Input: part model. Units: mm. Frame: model coordinates. A direction names the side the tool comes from. Give positions to 0.01 mm unless a question says otherwise; leave off trailing zeros. Loops run counter-clockwise (first coordinate to the right, second up) from the corner with the lowest first, then second, coordinate; pieces in that order, holes last. Notation, with made-up numbers: M -22,0 L 20,0 A23 cw 20,17 Z; hole C 0.25,-29 d5. An arc over 180 degrees is marked long. Answer as a JSON object with one key per item and string values. Group by question number.
```python
from build123d import *

# Parameters (mm, degrees)
F1_DEPTH = 5.08
F3_DEPTH = 25.4
F4_R     = 2.54
F5_R     = 1.524


with BuildPart() as f1:
    # F0 (on Top) → F1 (new body)
    with BuildSketch(Plane.XY):
        with BuildLine():
            ThreePointArc((-13.7862916745, 2.2581102419), (-1.1327853518, -13.9239971756), (13.97, 0))
            ThreePointArc((13.97, 0), (13.9239971756, 1.1327853518), (13.7862916745, 2.2581102419))
            ThreePointArc((13.7862916745, 2.2581102419), (9.0447526202, 10.646753028), (0, 13.97))
            ThreePointArc((0, 13.97), (-9.0447526202, 10.646753028), (-13.7862916745, 2.2581102419))
        make_face()
        with BuildLine():
            Line((-6.6675, 45.72), (-13.7862916745, 2.2581102419))
            ThreePointArc((-13.7862916745, 2.2581102419), (-9.0447526202, 10.646753028), (0, 13.97))
            Line((0, 13.97), (-1.5875, 13.97))
            Line((-1.5875, 13.97), (-1.5875, 45.72))
            Line((-1.5875, 45.72), (-6.6675, 45.72))
        make_face()
        with BuildLine():
            ThreePointArc((0, 13.97), (9.0447526202, 10.646753028), (13.7862916745, 2.2581102419))
            Line((13.7862916745, 2.2581102419), (6.6675, 45.72))
            Line((6.6675, 45.72), (1.5875, 45.72))
            Line((1.5875, 45.72), (1.5875, 13.97))
            Line((1.5875, 13.97), (0, 13.97))
        make_face()
    extrude(amount=F1_DEPTH)

    # F2 (on face) → F3 (cut)
    with BuildSketch(Plane.XY.offset(5.08)):
        with BuildLine():
            Line((-3.7422612851, 9.0346179484), (-1.9134612851, 9.0346179484))
            ThreePointArc((-1.9134612851, 9.0346179484), (-4.4421127462, 10.7242088375), (-5.0354181665, 7.741461067))
            Line((-5.0354181665, 7.741461067), (-3.7422612851, 9.0346179484))
        make_face()
        with BuildLine():
            ThreePointArc((-5.0354181665, 7.741461067), (-3.042409824, 7.3450270594), (-1.9134612851, 9.0346179484))
            Line((-1.9134612851, 9.0346179484), (-3.7422612851, 9.0346179484))
            Line((-3.7422612851, 9.0346179484), (-5.0354181665, 7.741461067))
        make_face()
        with BuildLine():
            Line((3.7422612851, 9.0346179484), (5.0354181665, 7.741461067))
            ThreePointArc((5.0354181665, 7.741461067), (5.4318521742, 8.3347664873), (5.5710612851, 9.0346179484))
            ThreePointArc((5.5710612851, 9.0346179484), (3.7422612851, 10.8634179484), (1.9134612851, 9.0346179484))
            Line((1.9134612851, 9.0346179484), (3.7422612851, 9.0346179484))
        make_face()
        with BuildLine():
            ThreePointArc((1.9134612851, 9.0346179484), (3.042409824, 7.3450270594), (5.0354181665, 7.741461067))
            Line((5.0354181665, 7.741461067), (3.7422612851, 9.0346179484))
            Line((3.7422612851, 9.0346179484), (1.9134612851, 9.0346179484))
        make_face()
        with BuildLine():
            Line((7.741461067, 5.0354181665), (9.0346179484, 3.7422612851))
            Line((9.0346179484, 3.7422612851), (9.0346179484, 1.9134612851))
            ThreePointArc((9.0346179484, 1.9134612851), (10.3277748299, 2.4491044037), (10.8634179484, 3.7422612851))
            ThreePointArc((10.8634179484, 3.7422612851), (9.7344694095, 5.4318521742), (7.741461067, 5.0354181665))
        make_face()
        with BuildLine():
            Line((9.0346179484, 1.9134612851), (9.0346179484, 3.7422612851))
            Line((9.0346179484, 3.7422612851), (7.741461067, 5.0354181665))
            ThreePointArc((7.741461067, 5.0354181665), (7.3450270594, 3.042409824), (9.0346179484, 1.9134612851))
        make_face()
        with BuildLine():
            ThreePointArc((10.8634179484, -3.7422612851), (10.3277748299, -2.4491044037), (9.0346179484, -1.9134612851))
            Line((9.0346179484, -1.9134612851), (9.0346179484, -3.7422612851))
            Line((9.0346179484, -3.7422612851), (7.741461067, -5.0354181665))
            ThreePointArc((7.741461067, -5.0354181665), (9.7344694095, -5.4318521742), (10.8634179484, -3.7422612851))
        make_face()
        with BuildLine():
            Line((9.0346179484, -3.7422612851), (9.0346179484, -1.9134612851))
            ThreePointArc((9.0346179484, -1.9134612851), (7.3450270594, -3.042409824), (7.741461067, -5.0354181665))
            Line((7.741461067, -5.0354181665), (9.0346179484, -3.7422612851))
        make_face()
        with BuildLine():
            ThreePointArc((5.5710612851, -9.0346179484), (5.4318521742, -8.3347664873), (5.0354181665, -7.741461067))
            Line((5.0354181665, -7.741461067), (3.7422612851, -9.0346179484))
            Line((3.7422612851, -9.0346179484), (1.9134612851, -9.0346179484))
            ThreePointArc((1.9134612851, -9.0346179484), (3.7422612851, -10.8634179484), (5.5710612851, -9.0346179484))
        make_face()
        with BuildLine():
            Line((3.7422612851, -9.0346179484), (5.0354181665, -7.741461067))
            ThreePointArc((5.0354181665, -7.741461067), (3.042409824, -7.3450270594), (1.9134612851, -9.0346179484))
            Line((1.9134612851, -9.0346179484), (3.7422612851, -9.0346179484))
        make_face()
        with BuildLine():
            ThreePointArc((-5.0354181665, -7.741461067), (-4.4421127462, -10.7242088375), (-1.9134612851, -9.0346179484))
            Line((-1.9134612851, -9.0346179484), (-3.7422612851, -9.0346179484))
            Line((-3.7422612851, -9.0346179484), (-5.0354181665, -7.741461067))
        make_face()
        with BuildLine():
            Line((-3.7422612851, -9.0346179484), (-1.9134612851, -9.0346179484))
            ThreePointArc((-1.9134612851, -9.0346179484), (-3.042409824, -7.3450270594), (-5.0354181665, -7.741461067))
            Line((-5.0354181665, -7.741461067), (-3.7422612851, -9.0346179484))
        make_face()
        with BuildLine():
            Line((-9.0346179484, -3.7422612851), (-7.741461067, -5.0354181665))
            ThreePointArc((-7.741461067, -5.0354181665), (-7.3450270594, -4.4421127462), (-7.2058179484, -3.7422612851))
            ThreePointArc((-7.2058179484, -3.7422612851), (-7.741461067, -2.4491044037), (-9.0346179484, -1.9134612851))
            Line((-9.0346179484, -1.9134612851), (-9.0346179484, -3.7422612851))
        make_face()
        with BuildLine():
            ThreePointArc((-9.0346179484, -1.9134612851), (-10.7242088375, -4.4421127462), (-7.741461067, -5.0354181665))
            Line((-7.741461067, -5.0354181665), (-9.0346179484, -3.7422612851))
            Line((-9.0346179484, -3.7422612851), (-9.0346179484, -1.9134612851))
        make_face()
        with BuildLine():
            Line((-9.0346179484, 3.7422612851), (-7.741461067, 5.0354181665))
            ThreePointArc((-7.741461067, 5.0354181665), (-10.7242088375, 4.4421127462), (-9.0346179484, 1.9134612851))
            Line((-9.0346179484, 1.9134612851), (-9.0346179484, 3.7422612851))
        make_face()
        with BuildLine():
            ThreePointArc((-7.2058179484, 3.7422612851), (-7.3450270594, 4.4421127462), (-7.741461067, 5.0354181665))
            Line((-7.741461067, 5.0354181665), (-9.0346179484, 3.7422612851))
            Line((-9.0346179484, 3.7422612851), (-9.0346179484, 1.9134612851))
            ThreePointArc((-9.0346179484, 1.9134612851), (-7.741461067, 2.4491044037), (-7.2058179484, 3.7422612851))
        make_face()
    extrude(amount=-F3_DEPTH, mode=Mode.SUBTRACT)

    # F4
    f4_edges = [f1.edges().sort_by_distance(p)[0] for p in [
        (1.5875, 45.72, 2.54),
        (-1.5875, 45.72, 2.54),
        (-6.6675, 45.72, 2.54),
        (6.6675, 45.72, 2.54),
    ]]
    fillet(f4_edges, radius=F4_R)

    # F5
    f5_edges = [f1.edges().sort_by_distance(p)[0] for p in [
        (-1.5875, 13.97, 2.54),
        (1.5875, 13.97, 2.54),
    ]]
    fillet(f5_edges, radius=F5_R)


solid = f1.part
```
1. Material intervals for L1, parallel to Y at x = -4.5, z = 2.2; L2, parallel to Y at x = 3.25, z = 2.65; L3, parallel to X at y = -2.5, z = 0.7, sorted ascending.
2. Section C-C (x = 3.25). Output: boundary loops of the cut face in (y, z).
3. Mould query, pull axis X, two halves, no side actions, for faces 3 (the cylindrical face through (2.351, 44.996, 2.576)), 4 (the flat face through (-10.354, 23.214, 2.504)), 5 (the cylindrical face through (6.17, 45.1, 2.58)). Classes: pulls with the +X half, pulls with the -X half, needs draft (parallel to the pull), parting line crosses it, or undercut.
4. Section D-D (y = 29). Output: boundary loops of the cut face in (x, z).
5. Section B-B (z = 2.4). Count the separate pieces of the cut face and the enclosed holes in it, then the cut area to 3 significant figures.
6. Section A-A (y = 16.5). Output: boundary loops of the cut face in (x, z).
7. Reachability of faces 1 (the flat face through (10.449, 22.635, 2.504)), 2 (the flat face through (-1.588, 29, 3)) from +Z, -Z, +X, -X, +Y, -Y: full face, straight path, thin tool, end or side. Return the list, or none.
8. First-contact query: P1, Ø2, axis at x = -9.03, y = 3.74, coming from the +Z side; P2, Ø2.5, axis at y = 23.5, z = 3, coming from the -X side; P3, Ø3, axis at y = 28.5, z = 2.5, coming from the -X side. Flat tips, straight axial feed; report the tip coordinate or a pass-through.
Geometry results:
{
 "1": {"L1": "-13.23 to -10.7, -7.37 to 7.37, 10.7 to 45.72", "L2": "-13.59 to -10.8, -7.27 to 7.27, 10.8 to 45.56", "L3": "-13.74 to -10.38, -7.69 to 7.69, 10.38 to 13.74"},
 "2": {"outline": "M -13.59,0 L -10.8,0 L -10.8,5.08 L -13.59,5.08 Z; M -7.27,0 L 7.27,0 L 7.27,5.08 L -7.27,5.08 Z; M 10.8,0 L 45.56,0 L 45.56,5.08 L 10.8,5.08 Z"},
 "3": {"face 3": "undercut", "face 4": "pulls with the -X half", "face 5": "pulls with the +X half"},
 "4": {"outline": "M -9.41,0 L -1.59,0 L -1.59,5.08 L -9.41,5.08 Z; M 1.59,0 L 9.41,0 L 9.41,5.08 L 1.59,5.08 Z"},
 "5": {"separate pieces": "1", "enclosed holes": "8", "area": "1,070 mm2"},
 "6": {"outline": "M -11.45,0 L -1.59,0 L -1.59,5.08 L -11.45,5.08 Z; M 1.59,0 L 11.45,0 L 11.45,5.08 L 1.59,5.08 Z"},
 "7": {"face 1": "+Z, -Z, +X, +Y", "face 2": "+Z, -Z, +Y"},
 "8": {"P1": "through", "P2": "x = -10.51", "P3": "x = -9.73"}
}
